```python
from build123d import *

# Parameters (mm, degrees)
SKETCH1_R               = 201.6125
BASE_EXTRUDE_DEPTH      = 15.875
CUT_EXTRUDE1_DEPTH      = 286.564731607
CUT_EXTRUDE1_DEPTH_BACK = 286.564731607
CIRPATTERN1_COUNT       = 20
CHAMFER1_SIZE           = 0.762


with BuildPart() as part:
    # Sketch1 → Base-Extrude (new body)
    with BuildSketch(Plane.XY):
        Circle(SKETCH1_R)
        with BuildLine():
            ThreePointArc((22.991911078, -137.795), (0, 139.7), (-22.991911078, -137.795))
            ThreePointArc((-22.991911078, -137.795), (0, -152.4), (22.991911078, -137.795))
        make_face(mode=Mode.SUBTRACT)
    extrude(amount=BASE_EXTRUDE_DEPTH)

    # Sketch7 → Cut-Extrude1 (cut, two sides: drawn at the far end of the back side and taken through both)
    with BuildSketch(Plane(origin=(0, 0, 0), x_dir=(0, 0, -1), z_dir=(1, 0, 0)).offset(-CUT_EXTRUDE1_DEPTH_BACK)):
        Polygon((-14.3002, 1056.882009862), (-14.3002, 214.087795121), (-14.3002, -214.538981202), (-14.3002, -1057.333195943), (-1699.888629482, -1057.333195943), (-1699.888629482, 1056.882009862), align=None)
    extrude(amount=CUT_EXTRUDE1_DEPTH + CUT_EXTRUDE1_DEPTH_BACK, mode=Mode.SUBTRACT)

    # Sketch9 → 5_8 _0.625_ Diameter Hole1 (revolve, cut)
    with BuildSketch(Plane(origin=(181.882807921, 28.807406737, 14.3002), x_dir=(0, -1, 0), z_dir=(1, 0, 0))):
        Polygon((0, 0), (0, 14.3002), (8.382, 14.3002), (8.1915, 13.840292316), (8.1915, 0.459907684), (8.382, 0), align=None)
    f_5_8_0_625_diameter_hole1 = revolve(axis=Axis((181.882807921, 28.807406737, 20.6502), (0, 0, -1)), mode=Mode.SUBTRACT)

    # CirPattern1: 5_8 _0.625_ Diameter Hole1 ×20 about axis
    cirpattern1_axis = Axis((0, 0, 0), (0, 0, 1))
    for i in range(1, CIRPATTERN1_COUNT):
        add(f_5_8_0_625_diameter_hole1.rotate(cirpattern1_axis, i * 360 / CIRPATTERN1_COUNT), mode=Mode.SUBTRACT)

    # Chamfer1
    chamfer1_edges = [part.edges().sort_by_distance(p)[0] for p in [
        (-201.6125, 0, 14.3002),
        (-201.6125, 0, 0),
    ]]
    chamfer(chamfer1_edges, length=CHAMFER1_SIZE)


solid = part.part
```
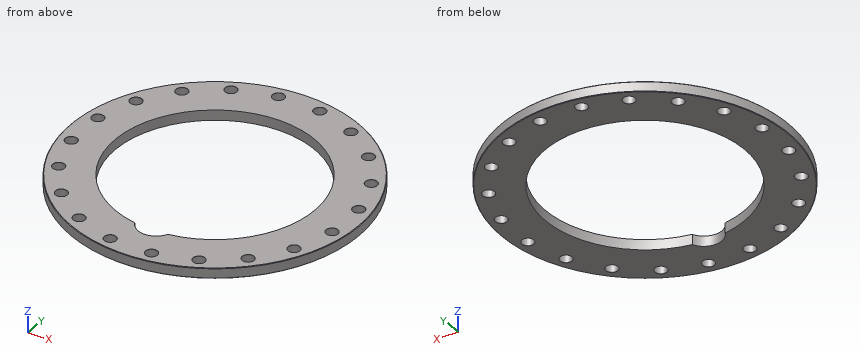
Work out the finished part from the listing and answer in its coordinate system (mm). Coordinates: 2 decimals unless noted, no trailing zeros. Loops run counter-clockwise (first coordinate to the right, second up) from the corner with the lowest first, then second, coordinate; pieces in that order, holes last. Notation, with made-up numbers: (-20, -2.75) - (38, -2.75) arc R8 ccw to (38, 12.25) - close; hole circle Ø11 at (-3.5, 4). An arc over 180 degrees is marked (long way). Use a Markdown table: item, result.
Item 1: Find section C-C, the plane z = 5.25. State how many separate pieces and enclosed holes the cut face has, and give its area (3 significant figures).
Evaluation:
| item | result |
|---|---|
| separate pieces | 1 |
| enclosed holes | 21 |
| area | 61,700 mm2 |
Item 2: Given pin 1 Ø3 at (y, z) = (-148.5, 9.5) entering from +X; pin 2 Ø10 at (x, y) = (-164.08, -83.6) entering from +Z (3 decimals); pin 3 Ø21.5 at (x, y) = (-130.21, -130.21) entering from -Z; pin 4 Ø8 at (y, z) = (-89.5, 5.5) entering from -X, each flat-ended and moving along its own axis, determine where each tip first touches the part or whether it passes through.
Evaluation:
| item | result |
|---|---|
| pin 1 | stops at x = 137.98 |
| pin 2 | passes through |
| pin 3 | stops at z = 0 |
| pin 4 | stops at x = -182.59 |
Item 3: Find section A-A, the plane y = 0. Determine the outline of the cut face in (x, z).
Evaluation:
| item | result |
|---|---|
| outline | (-201.61, 0.76) - (-200.85, 0) - (-139.7, 0) - (-139.7, 14.3) - (-200.85, 14.3) - (-201.61, 13.54) - close; (139.7, 0) - (200.85, 0) - (201.61, 0.76) - (201.61, 13.54) - (200.85, 14.3) - (139.7, 14.3) - close |
Item 4: Consider probe 1 along X at (y, z) = (80, 12.25); probe 2 along X at (y, z) = (-36, 2); probe 3 along Y at (x, z) = (-126, 5.25). Determine where each line is inside the solid, lowest interval first. Write a range as from..to.
Evaluation:
| item | result |
|---|---|
| probe 1 | x = -185.06..-171.44, -156.72..-114.53, 114.53..156.72, 171.44..185.06 |
| probe 2 | x = -198.37..-185.8, -177.96..-134.98, 134.98..177.96, 185.8..198.37 |
| probe 3 | y = -157.39..-137.24, -123.19..-60.33, 60.33..123.19, 137.24..157.39 |
Item 5: Find section B-B, the plane x = 0. Determine the outline of the cut face in (y, z).
Evaluation:
| item | result |
|---|---|
| outline | (-201.61, 0.76) - (-200.85, 0) - (-152.4, 0) - (-152.4, 14.3) - (-200.85, 14.3) - (-201.61, 13.54) - close; (139.7, 0) - (200.85, 0) - (201.61, 0.76) - (201.61, 13.54) - (200.85, 14.3) - (139.7, 14.3) - close |
